Geometry check sheet. Reference: the model listing, model coordinates, mm. A direction names the side the tool comes from. Coordinates: 2 decimals unless noted, no trailing zeros. Write each loop counter-clockwise with the first axis right and the second up, starting at its lowest first coordinate (ties: lowest second). Pieces come first, ordered by that corner, then holes. Notation, with made-up numbers: M 49.5,37 L 54.5,37 A31 ccw 54.5,72 Z; hole C -7.5,86 d2. An arc over 180 degrees is marked long. Put each result on its own line as item: value. Start each with the question number.
1) Cross-section at A-A on y = -18.5. Count the separate pieces of the cut face and the enclosed holes in it, plus the area to 3 significant figures.
2) Set-up check for faces 1 (the flat face through (10, -10, 26)), 2 (the flat face through (15.67, -5.42, -18.27)), 3 (the flat face through (-26, -10, -10)): record each of +Z, -Z, +X, -X, +Y, -Y from which the full face is reachable in a straight line by a thin tool's end or side.
3) Gauge pin test, flat ends, axial feed: pin 1 (1.8 mm diameter, centred on x = -27, y = -9.5, fed in from +Z); pin 2 (12 mm diameter, centred on x = -20, z = 23.5, fed in from +Y); pin 3 (5 mm diameter, centred on x = 14, y = -16, fed in from -Z); pin 4 (1.8 mm diameter, centred on x = 27, y = -12.5, fed in from -Z). Record the tip position at first contact, or that the pin passes through.
4) Mould release check, pull along Y, two halves, no side actions. Record for faces 4 (the cylindrical face through (-12.558, -5.254, 12.854)), 5 (the cylindrical face through (-15.96, -9.86, -15.86)), 6 (the flat face through (13, -20, 0)): released by +Y, released by -Y, zero draft, split by the parting line, or undercut.
5) Scan lines: line 1 along Z through (x, y) = (0, -15); line 2 along X through (y, z) = (-18, -2.5); line 3 along Z through (x, y) = (-22, -13). Record each from-to range of solid material in increasing order.
6) Cross-section at C-C on z = -1.5. Record the cut outline in (x, y), plus the area to 3 significant figures.
7) Cross-section at B-B on x = 0. Record the cut outline in (y, z), plus the area to 3 significant figures.
from build123d import *

# Parameters (mm, degrees)
F0_R      = 22.5
F0_R_2    = 12.69
F1_DEPTH  = 20
F3_DEPTH  = 20
F5_R      = 4
F6_DEPTH  = 52.7
F8_DEPTH  = 20
F9_R      = 5
F10_R     = 4.75
F11_DEPTH = 55.8


with BuildPart() as f1:
    # F0 (on Front) → F1 (new body)
    with BuildSketch(Plane.XZ):
        Circle(F0_R)
        Circle(F0_R_2, mode=Mode.SUBTRACT)
    extrude(amount=F1_DEPTH)

    # F2 (on Front) → F3 (join)
    with BuildSketch(Plane.XZ):
        with BuildLine():
            Line((10, 14.3614066163), (10, 28.2842712475))
            ThreePointArc((10, 28.2842712475), (0, 30), (-10, 28.2842712475))
            Line((-10, 28.2842712475), (-10, 14.3614066163))
            ThreePointArc((-10, 14.3614066163), (0, 17.5), (10, 14.3614066163))
        make_face()
        with BuildLine():
            Line((-14.3614066163, 10), (-28.2842712475, 10))
            ThreePointArc((-28.2842712475, 10), (-30, 0), (-28.2842712475, -10))
            Line((-28.2842712475, -10), (-14.3614066163, -10))
            ThreePointArc((-14.3614066163, -10), (-17.5, 0), (-14.3614066163, 10))
        make_face()
        with BuildLine():
            ThreePointArc((28.2842712475, -10), (30, 0), (28.2842712475, 10))
            Line((28.2842712475, 10), (14.3614066163, 10))
            ThreePointArc((14.3614066163, 10), (17.5, 0), (14.3614066163, -10))
            Line((14.3614066163, -10), (28.2842712475, -10))
        make_face()
        with BuildLine():
            Line((-10, -14.3614066163), (-10, -28.2842712475))
            ThreePointArc((-10, -28.2842712475), (0, -30), (10, -28.2842712475))
            Line((10, -28.2842712475), (10, -14.3614066163))
            ThreePointArc((10, -14.3614066163), (0, -17.5), (-10, -14.3614066163))
        make_face()
    extrude(amount=F3_DEPTH)

    # F5 (on Front) → F6 (cut)
    with BuildSketch(Plane.XZ):
        with Locations((0, 22)):
            Circle(F5_R)
        with Locations((0, -22)):
            Circle(F5_R)
        with Locations((22, 0)):
            Circle(F5_R)
        with Locations((-22, 0)):
            Circle(F5_R)
    extrude(amount=F6_DEPTH, mode=Mode.SUBTRACT)

    # F7 (on Front) → F8 (join)
    with BuildSketch(Plane.XZ):
        with BuildLine():
            Line((-7, 26.941125497), (-26.941125497, 7))
            Line((-26.941125497, 7), (-13.2664991614, 7))
            ThreePointArc((-13.2664991614, 7), (-10.6066017178, 10.6066017178), (-7, 13.2664991614))
            Line((-7, 13.2664991614), (-7, 26.941125497))
        make_face()
        with BuildLine():
            Line((26.941125497, -7), (13.2664991614, -7))
            ThreePointArc((13.2664991614, -7), (10.6066017178, -10.6066017178), (7, -13.2664991614))
            Line((7, -13.2664991614), (7, -26.941125497))
            Line((7, -26.941125497), (26.941125497, -7))
        make_face()
    extrude(amount=F8_DEPTH)

    # F9
    f9_edges = [f1.edges().sort_by_distance(p)[0] for p in [
        (10, -10, 20.155644),
        (20.155644, -10, 10),
        (-10, -10, -20.155644),
        (-20.155644, -10, -10),
        (-10, -10, 23.941125),
        (-23.941125, -10, 10),
        (23.941125, -10, -10),
        (10, -10, -23.941125),
    ]]
    fillet(f9_edges, radius=F9_R)

    # F10 (on face) → F11 (cut, symmetric)
    with BuildSketch(Plane(origin=(-16.9705627485, 0, 16.9705627485), x_dir=(0, -1, 0), z_dir=(-0.7071067812, 0, 0.7071067812))):
        with Locations((9.9991243333, 0)):
            Circle(F10_R)
    extrude(amount=F11_DEPTH, both=True, mode=Mode.SUBTRACT)


solid = f1.part
Answer key:
1. separate pieces: 1
1. enclosed holes: 5
1. area: 1,580 mm²
2. face 1: +Z, +X, +Y, -Y
2. face 2: -Z, +X, +Y, -Y
2. face 3: -Z, -X, +Y, -Y
3. pin 1: stops at z = 10
3. pin 2: passes through
3. pin 3: stops at z = -22.44
3. pin 4: stops at z = -10
4. face 4: undercut
4. face 5: zero draft
4. face 6: released by -Y
5. line 1: z = -30 to -26, -18 to -12.69, 12.69 to 18, 26 to 30
5. line 2: x = -29.9 to -25.12, -18.88 to -12.44, 12.44 to 18.88, 25.12 to 29.9
5. line 3: z = -10.11 to -4, 4 to 11.94
6. outline: M -29.96,-20 L -25.71,-20 L -25.71,0 L -29.96,0 Z; M -18.29,-20 L -12.6,-20 L -12.6,0 L -18.29,0 Z; M 12.6,-20 L 18.29,-20 L 18.29,0 L 12.6,0 Z; M 25.71,-20 L 29.96,-20 L 29.96,0 L 25.71,0 Z
6. area: 398 mm²
7. outline: M -20,-30 L 0,-30 L 0,-26 L -20,-26 Z; M -20,-18 L 0,-18 L 0,-12.69 L -20,-12.69 Z; M -20,12.69 L 0,12.69 L 0,18 L -20,18 Z; M -20,26 L 0,26 L 0,30 L -20,30 Z
7. area: 372 mm²
